Print and shaded views of the part. All mm, measured from the part's lowest x, y and z. Round coordinates to 2 decimals unless told otherwise and drop trailing zeros. Loops run counter-clockwise (first coordinate to the right, second up) from the corner with the lowest first, then second, coordinate; pieces in that order, holes last. Notation, with made-up numbers: (15, 83.25) - (29, 83.25) arc R16 cw to (29, 105.25) - close; hole circle Ø3 at (45.25, 44). An arc over 180 degrees is marked (long way). Answer as a JSON object with one key per item and string values.
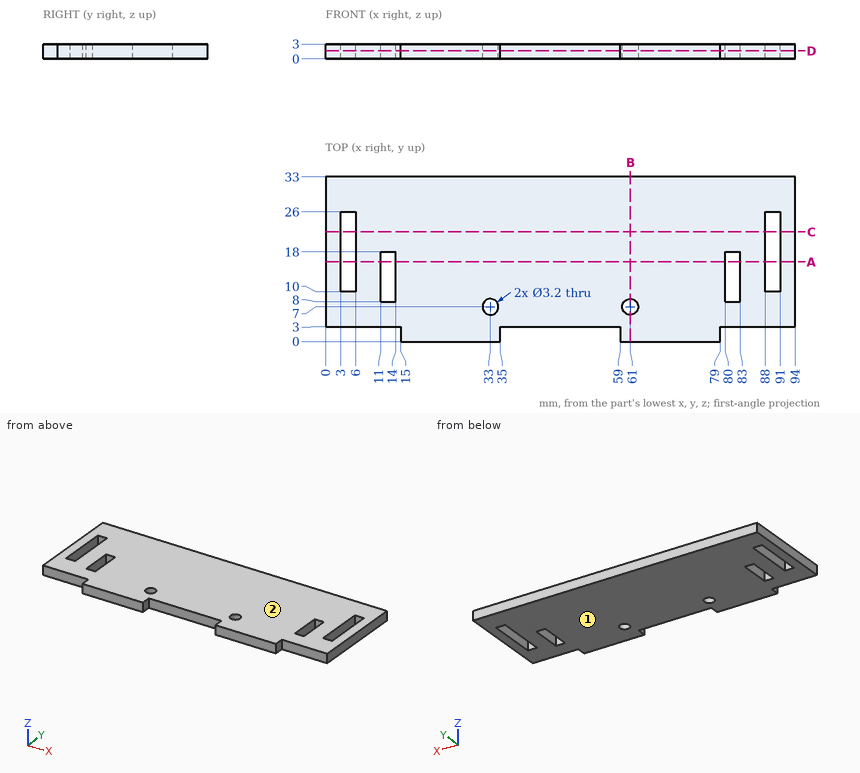
1) Probe probe 1 along X at (y, z) = (24, 0.7); probe 2 along X at (y, z) = (17, 2.4); probe 3 along Y at (x, z) = (33, 1.8). List the from-to ranges inside material, lowest first.
Values follow:
{"probe 1": "0 to 3, 6 to 88, 91 to 94", "probe 2": "0 to 3, 6 to 11, 14 to 80, 83 to 88, 91 to 94", "probe 3": "0 to 5.4, 8.6 to 33"}
2) Drop flat-ended pins along their axis: P1, Ø1.5, axis at x = 4.5, z = 1.5, coming from the -Y side; P2, Ø2.5, axis at x = 61, y = 7, coming from the -Z side. Give the stop position or say it passes through.
Values follow:
{"P1": "y = 3", "P2": "through"}
3) Two-plate mould, pull along Z, no slides. Class the marked faces 1 and 2: pulls with the +Z half, pulls with the -Z half, needs draft (parallel to the pull), parting line crosses it, or undercut.
Values follow:
{"face 1": "pulls with the -Z half", "face 2": "pulls with the +Z half"}
4) Slice it at A-A on y = 16. List the corners of the cut face in (x, z).
Values follow:
{"outline": "(0, 0) - (3, 0) - (3, 3) - (0, 3) - close; (6, 0) - (11, 0) - (11, 3) - (6, 3) - close; (14, 0) - (80, 0) - (80, 3) - (14, 3) - close; (83, 0) - (88, 0) - (88, 3) - (83, 3) - close; (91, 0) - (94, 0) - (94, 3) - (91, 3) - close"}
5) Slice it at B-B on x = 61. List the corners of the cut face in (y, z), then the cut area to 3 significant figures.
Values follow:
{"outline": "(0, 0) - (5.4, 0) - (5.4, 3) - (0, 3) - close; (8.6, 0) - (33, 0) - (33, 3) - (8.6, 3) - close", "area": "89.4 mm²"}
6) Slice it at C-C on y = 22. List the corners of the cut face in (x, z), then the cut area to 3 significant figures.
Values follow:
{"outline": "(0, 0) - (3, 0) - (3, 3) - (0, 3) - close; (6, 0) - (88, 0) - (88, 3) - (6, 3) - close; (91, 0) - (94, 0) - (94, 3) - (91, 3) - close", "area": "264 mm²"}
7) Slice it at D-D on z = 1.6. Count the separate pieces of the cut face and the enclosed holes in it, then the cut area to 3 significant figures.
Values follow:
{"separate pieces": "1", "enclosed holes": "6", "area": "2,770 mm²"}
